Can you work these out from the model? Positions are in its coordinate system, mm. Face numbers are marked on the shaded views. A direction names the side the tool comes from. Coordinates: 2 decimals unless noted, no trailing zeros. Order: outer loops, then holes, each group sorted by start corner. A loop starts at its lowest first (then second) coordinate and runs counter-clockwise, first axis right, second up. Notation, with made-up numbers: (12, 0) -> (52, 0) arc R20 cw to (52, 29) -> close; hole circle Ø1 at (2.25, 34.5). An arc over 180 degrees is marked (long way). Use a Markdown table: item, result. Add a question column.
1. We'd pull the mould along X, two halves only. Please class the marked faces 1, 2 and 3: pulls with the +X half, pulls with the -X half, needs draft (parallel to the pull), parting line crosses it, or undercut.
2. For pin 1 Ø4 at (y, z) = (5.5, 5) entering from +X; pin 2 Ø1.5 at (x, y) = (-0.5, -0.5) entering from +Z; pin 3 Ø4 at (y, z) = (-4, 2) entering from +X, each with a flat end and sliding along its axis, tell me the tip position at first contact or that it passes through.
3. Suppose I cut it at D-D, the plane z = 1.75. List the corners of the cut face in (x, y) for me.
4. Suppose I cut it at C-C, the plane z = 4.5. List the corners of the cut face in (x, y) for me.
5. If I drill on line 1 along Y through (x, z) = (0, 5.65); line 2 along Z through (x, y) = (9, 3.5); line 3 along Y through (x, z) = (-2.25, 5.5), over which ranges is the centre line in solid material (lowest first)? Write a range as from..to.
6. Suppose I cut it at A-A, the plane y = 0. List the corners of the cut face in (x, z) for me, then the cut area to 3 significant figures.
7. For the marked faces 4 and 5, which set-ups out of +Z, -Z, +X, -X, +Y, -Y let a thin tool reach every point of the face, with its end or its side?
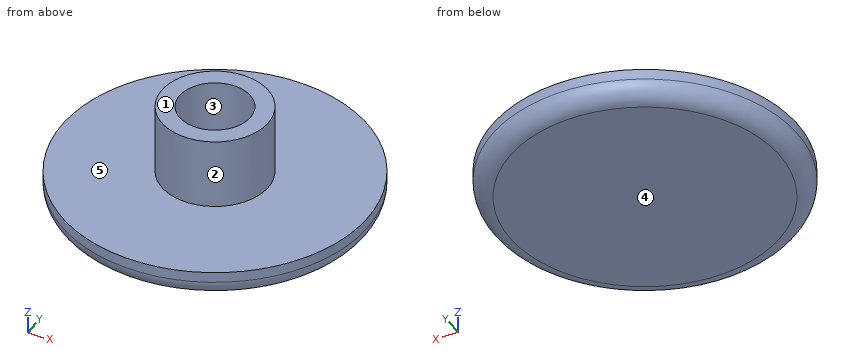
```python
from build123d import *

# Parameters (mm, degrees)
F0_R     = 10.922
F1_DEPTH = 2.032
F2_R     = 3.81
F3_DEPTH = 5.08
F4_R     = 2.54
F5_DEPTH = 5.08
F6_R     = 1.27


with BuildPart() as f1:
    # F0 (on Top) → F1 (new body)
    with BuildSketch(Plane.XY):
        Circle(F0_R)
    extrude(amount=F1_DEPTH)

    # F2 (on face) → F3 (join)
    with BuildSketch(Plane.XY.offset(2.032)):
        Circle(F2_R)
    extrude(amount=F3_DEPTH)

    # F4 (on face) → F5 (cut, through all)
    with BuildSketch(Plane.XY.offset(7.112)):
        Circle(F4_R)
    extrude(amount=-F5_DEPTH, mode=Mode.SUBTRACT)

    # F6
    f6_edges = [f1.edges().sort_by_distance(p)[0] for p in [
        (-10.922, 0, 0),
    ]]
    fillet(f6_edges, radius=F6_R)


solid = f1.part
```
Worked out:
| question | item | result |
|---|---|---|
| 1 | face 1 | needs draft |
| 1 | face 2 | parting line crosses it |
| 1 | face 3 | undercut |
| 2 | pin 1 | stops at x = 1.51 |
| 2 | pin 2 | stops at z = 2.03 |
| 2 | pin 3 | stops at x = 10.74 |
| 3 | outline | circle Ø21.84 at (0, 0) |
| 4 | outline | circle Ø7.62 at (0, 0); hole circle Ø5.08 at (0, 0) |
| 5 | line 1 | y = -3.81..-2.54, 2.54..3.81 |
| 5 | line 2 | z = 0..2.03 |
| 5 | line 3 | y = -3.07..-1.18, 1.18..3.07 |
| 6 | outline | (-10.92, 1.27) arc R1.27 ccw to (-9.65, 0) -> (9.65, 0) arc R1.27 ccw to (10.92, 1.27) -> (10.92, 2.03) -> (3.81, 2.03) -> (3.81, 7.11) -> (2.54, 7.11) -> (2.54, 2.03) -> (-2.54, 2.03) -> (-2.54, 7.11) -> (-3.81, 7.11) -> (-3.81, 2.03) -> (-10.92, 2.03) -> close |
| 6 | area | 56.6 mm² |
| 7 | face 4 | -Z, +X, -X, +Y, -Y |
| 7 | face 5 | +Z |
